from build123d import *

# Parameters (mm, degrees)
F0_R     = 12.7
F1_DEPTH = 25.4
F2_W     = 101.6
F2_H     = 5.08
F3_DEPTH = 2.54
F4_R     = 1.905
F5_DEPTH = 15.241
F6_W     = 6.35
F6_H     = 2.54
F7_DEPTH = 15.241


with BuildPart() as f1:
    # F0 (on Right) → F1 (new body)
    with BuildSketch(Plane.YZ):
        Circle(F0_R)
    extrude(amount=F1_DEPTH)

    # F2 (on Top) → F3 (join, symmetric)
    with BuildSketch(Plane.XY):
        with Locations((76.2, 0)):
            Rectangle(F2_W, F2_H)
    extrude(amount=F3_DEPTH, both=True)

    # F4 (on face) → F5 (cut, through all)
    with BuildSketch(Plane.XZ.offset(2.54)):
        with Locations((124.46, 0)):
            Circle(F4_R)
    extrude(amount=-F5_DEPTH, mode=Mode.SUBTRACT)

    # F6 (on face) → F7 (cut, through all)
    with BuildSketch(Plane.XY.offset(2.54)):
        with Locations((123.825, 0)):
            Rectangle(F6_W, F6_H)
    extrude(amount=-F7_DEPTH, mode=Mode.SUBTRACT)


solid = f1.part
Design review of the part built by this model. Coordinates are the model's own, in mm. A direction names the side the tool comes from. Give positions to 0.01 mm unless a question says otherwise; leave off trailing zeros. Write each loop counter-clockwise with the first axis right and the second up, starting at its lowest first coordinate (ties: lowest second). Pieces come first, ordered by that corner, then holes. Notation, with made-up numbers: M -38,4 L 1,4 A34 cw 1,38 Z; hole C -37.75,56 d5. An arc over 180 degrees is marked long. Return JSON: item names as keys, results as strings. Group by question number.
Item 1: Take a section at C-C (y = 0). Give the boundary of the cut face in (x, z), plus the area to 3 significant figures.
Item 2: The part is to be moulded in two halves that separate along Z. For faces 1 (the cylindrical face through (122.557, 1.896, 0.084)), 2 (the flat face through (122, -1.27, 0)), 3 (the flat face through (75, 0, 2.54)), say which applies: pulls with the +Z half, pulls with the -Z half, needs draft (parallel to the pull), parting line crosses it, or undercut.
Item 3: Clearance check with flat-ended pins moving along their axes: pin 1 Ø6 at (x, z) = (124.46, 0) entering from +Y; pin 2 Ø2 at (y, z) = (0, 1) entering from +X; pin 3 Ø4 at (x, y) = (69.5, 0) entering from +Z. State where each tip first meets the part, or that it passes through.
Item 4: Take a section at B-B (z = 0). Give the boundary of the cut face in (x, y) (3 decimals), plus the area to 3 significant figures.
Item 5: Take a section at A-A (x = 124.46). Give the boundary of the cut face in (y, z) (3 decimals).
Item 6: Take a section at D-D (y = -7.75). Give the boundary of the cut face in (x, z).
Item 7: Wall thickness on line 1 along Z through (x, y) = (124.46, -1.7) (3 decimals); line 2 along X through (y, z) = (9.5, 1.75); line 3 along Y through (x, z) = (91.5, -0.5): over which ranges is each line inside the solid? List them lowest first.
Item 8: Tool access review of faces 4 (the flat face through (122, 1.27, 0)), 5 (the flat face through (75, 2.54, 0)), 6 (the flat face through (75, -2.54, 0)): name each direction out of +Z, -Z, +X, -X, +Y, -Y from which nothing blocks a thin tool from reaching the whole face with its end or side.
Return value:
{
 "1": {"outline": "M 0,-12.7 L 25.4,-12.7 L 25.4,-2.54 L 120.65,-2.54 L 120.65,2.54 L 25.4,2.54 L 25.4,12.7 L 0,12.7 Z", "area": "1,130 mm2"},
 "2": {"face 1": "undercut", "face 2": "needs draft", "face 3": "pulls with the +Z half"},
 "3": {"pin 1": "stops at y = 2.54", "pin 2": "stops at x = 120.65", "pin 3": "stops at z = 2.54"},
 "4": {"outline": "M 0,-12.7 L 25.4,-12.7 L 25.4,-2.54 L 122.555,-2.54 L 122.555,-1.27 L 120.65,-1.27 L 120.65,1.27 L 122.555,1.27 L 122.555,2.54 L 25.4,2.54 L 25.4,12.7 L 0,12.7 Z; M 126.365,-2.54 L 127,-2.54 L 127,-1.27 L 126.365,-1.27 Z; M 126.365,1.27 L 127,1.27 L 127,2.54 L 126.365,2.54 Z", "area": "1,140 mm2"},
 "5": {"outline": "M -2.54,-2.54 L -1.27,-2.54 L -1.27,-1.905 L -2.54,-1.905 Z; M -2.54,1.905 L -1.27,1.905 L -1.27,2.54 L -2.54,2.54 Z; M 1.27,-2.54 L 2.54,-2.54 L 2.54,-1.905 L 1.27,-1.905 Z; M 1.27,1.905 L 2.54,1.905 L 2.54,2.54 L 1.27,2.54 Z"},
 "6": {"outline": "M 0,-10.06 L 25.4,-10.06 L 25.4,10.06 L 0,10.06 Z"},
 "7": {"line 1": "z = -2.54 to -1.905, 1.905 to 2.54", "line 2": "x = 0 to 25.4", "line 3": "y = -2.54 to 2.54"},
 "8": {"face 4": "+Z, -Z, +X", "face 5": "+Z, -Z, +X, +Y", "face 6": "+Z, -Z, +X, -Y"}
}
